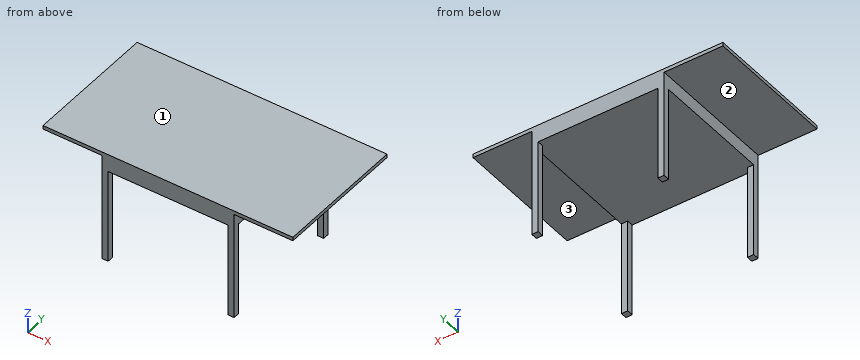
from build123d import *

# Parameters (mm, degrees)
SKETCH_W           = 1700
SKETCH_H           = 900
PAD_DEPTH          = 25
SKETCH001_W        = 900
SKETCH001_H        = 900
PAD001_DEPTH       = 95
SKETCH002_W        = 43
SKETCH002_H        = 43
PAD002_DEPTH       = 640
POLARPATTERN_COUNT = 4


with BuildPart() as part:
    # Sketch → Pad (new body)
    with BuildSketch(Plane.XY):
        Rectangle(SKETCH_W, SKETCH_H)
    extrude(amount=PAD_DEPTH)

    # Sketch001 (on Face5 of Pad) → Pad001 (join)
    with BuildSketch(Plane(origin=(0, 0, 0), x_dir=(1, 0, 0), z_dir=(0, 0, -1))):
        Rectangle(SKETCH001_W, SKETCH001_H)
    extrude(amount=PAD001_DEPTH)

    # Sketch002 (on Face11 of Pad001) → Pad002 (join)
    with BuildSketch(Plane(origin=(0, 0, -95), x_dir=(1, 0, 0), z_dir=(0, 0, -1))):
        with Locations((-428.5, -428.5)):
            Rectangle(SKETCH002_W, SKETCH002_H)
    pad002 = extrude(amount=PAD002_DEPTH)

    # PolarPattern: Pad002 ×4 about axis
    polarpattern_axis = Axis((0, 0, -95), (0, 0, -1))
    for i in range(1, POLARPATTERN_COUNT):
        add(pad002.rotate(polarpattern_axis, i * 360 / POLARPATTERN_COUNT))


solid = part.part
Part model, mm, in its own coordinate system. Face numbers are marked on the shaded views. A direction names the side the tool comes from. Give positions to 0.01 mm unless a question says otherwise; leave off trailing zeros. Write each loop counter-clockwise with the first axis right and the second up, starting at its lowest first coordinate (ties: lowest second). Pieces come first, ordered by that corner, then holes.
1) Which spindle directions (+Z, -Z, +X, -X, +Y, -Y) get a long thin tool onto all of the face, cutting with end or side? Do the marked faces 1, 2 and 3. Say none if no direction does.
Resolved:
face 1: +Z, +X, -X, +Y, -Y
face 2: -Z, -X, +Y, -Y
face 3: -Z, +X, +Y, -Y
2) Cut at A-A on z = -200. Write the cut outline in (x, y).
Resolved:
outline: (-450, -450) - (-407, -450) - (-407, -407) - (-450, -407) - close; (-450, 407) - (-407, 407) - (-407, 450) - (-450, 450) - close; (407, -450) - (450, -450) - (450, -407) - (407, -407) - close; (407, 407) - (450, 407) - (450, 450) - (407, 450) - close
3) Pin check, flat tips, straight feed: pin 1 (1.5 mm diameter, centred on x = -469.5, y = -336, fed in from -Z); pin 2 (21.5 mm diameter, centred on y = -420.5, z = -436.5, fed in from -X); pin 3 (6 mm diameter, centred on y = -254.5, z = -51.5, fed in from +X). Stop position of each tip, or through.
Resolved:
pin 1: stops at z = 0
pin 2: stops at x = -450
pin 3: stops at x = 450
4) Cut at B-B on y = 384.5. Write the cut outline in (x, z), then the cut area to 3 significant figures.
Resolved:
outline: (-850, 0) - (-450, 0) - (-450, -95) - (450, -95) - (450, 0) - (850, 0) - (850, 25) - (-850, 25) - close
area: 128,000 mm2
5) Cut at C-C on x = 132. Write the cut outline in (y, z), then the cut area to 3 significant figures.
Resolved:
outline: (-450, -95) - (450, -95) - (450, 25) - (-450, 25) - close
area: 108,000 mm2
6) Probe L1, parallel to Y at x = -438.5, z = -422; L2, parallel to Z at x = 237.5, y = -278.5; L3, parallel to X at y = 95, z = -21. List the from-to ranges inside material, lowest first.
Resolved:
L1: y = -450 to -407, 407 to 450
L2: z = -95 to 25
L3: x = -450 to 450
7) Cut at D-D on z = -70. Write the cut outline in (x, y).
Resolved:
outline: (-450, -450) - (450, -450) - (450, 450) - (-450, 450) - close
